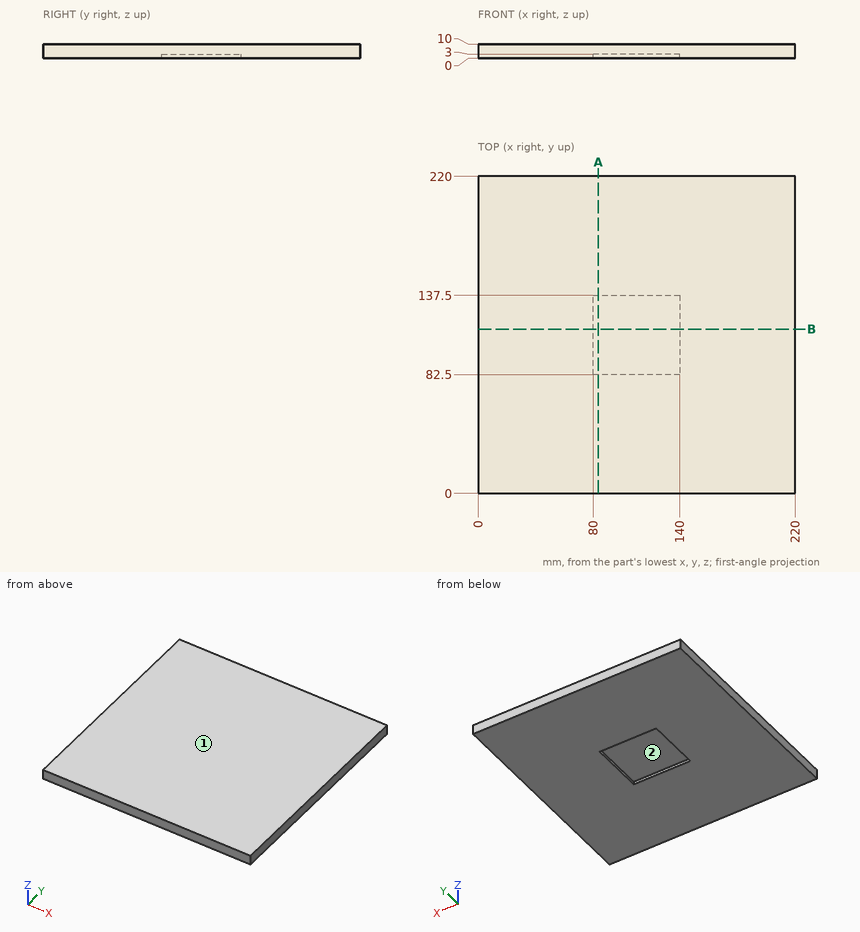
Job drawing, mm, ordinate dimensions from the low corner. One solid piece. Coordinates: 2 decimals unless noted, no trailing zeros. Write each loop counter-clockwise with the first axis right and the second up, starting at its lowest first coordinate (ties: lowest second). Pieces come first, ordered by that corner, then holes.
Item 1: Slice it at A-A (x = 83.5). Write the cut outline in (y, z).
Item 2: Mould opens along X. For the marked faces 1 and 2 say: released by +X, released by -X, zero draft, split by the parting line, or undercut.
Item 3: Probe line 1 (X direction, y = 85, z = 1.5). List the from-to ranges inside material, lowest first.
Item 4: Slice it at B-B (y = 114). Write the cut outline in (x, z), and give its area (3 significant figures).
Item 5: Pin check, flat tip, straight feed: pin 1 (1.5 mm diameter, centred on x = 134, y = 104, fed in from -Z). Stop position of the tip, or through.
Results found:
1. outline: (0, 0) - (82.5, 0) - (82.5, 3) - (137.5, 3) - (137.5, 0) - (220, 0) - (220, 10) - (0, 10) - close
2. face 1: zero draft
2. face 2: undercut
3. line 1: x = 0 to 80, 140 to 220
4. outline: (0, 0) - (80, 0) - (80, 3) - (140, 3) - (140, 0) - (220, 0) - (220, 10) - (0, 10) - close
4. area: 2,020 mm2
5. pin 1: stops at z = 3
